Input: part model. Units: mm. Frame: model coordinates. A direction names the side the tool comes from. Coordinates: 2 decimals unless noted, no trailing zeros. Loops run counter-clockwise (first coordinate to the right, second up) from the corner with the lowest first, then second, coordinate; pieces in that order, holes last. Notation, with made-up numbers: (86.25, 21) - (93.25, 21) arc R16 cw to (93.25, 34) - close; hole circle Ø8 at (-35.75, -8.75). An arc over 180 degrees is marked (long way). Use a Markdown table: item, result. Add a question column.
1. Access query for faces 4 (the face through (35.5, -12.7, -14.9)), 5 (the face through (-38.487, 5.15, 5.616)), 6 (the face through (-7.555, -0.992, -38.486)). Directions: +Z, -Z, +X, -X, +Y, -Y. A direction counts if a zero-diameter tool reaches every point of the face in a straight line with its end or side. Return the directions, or none.
2. Draft query along Z for faces 1 (the face through (35.5, 12.7, -14.9)), 2 (the face through (11.44, -0.18, 36.34)), 3 (the face through (11.92, 0.18, 37.84)). Return one class per face: released by +Z, released by -Z, zero draft, split by the parting line, or undercut.
3. Contact query for flat-ended pins moving along their axis: P1, Ø6, axis at y = 1.5, z = -30.5, coming from the -X side; P2, Ø4, axis at x = -21, z = -28.5, coming from the +Y side; P3, Ø12, axis at x = -12, y = 9, coming from the -Z side; P4, Ø3, axis at x = -7, y = 9, coming from the +Z side. Output: stop coordinate, or through.
4. Section query B-B on z = 0. Return the cut outline in (x, y).
5. Ray query, L1, parallel to Y at x = -39, z = 0; L2, parallel to Z at x = -2.5, y = -8.75; L3, parallel to X at y = -3.75, z = 18. Return the intervals inside material, ascending. Write a range as [from, to].
6. Section query D-D on x = 14. Return the cut outline in (y, z), then the cut area to 3 significant figures.
7. Section query A-A on x = 0. Return the cut outline in (y, z).
8. Section query C-C on y = 0. Return the cut outline in (x, z), then the cut area to 3 significant figures.
```python
from build123d import *

# Parameters (mm, degrees)
SKETCH1_R           = 39.6748
SKETCH1_R_2         = 38.1
BOSS_EXTRUDE1_DEPTH = 12.7
SKETCH2_R           = 7.62
CUT_EXTRUDE1_DEPTH  = 58.527988928
SKETCH3_R           = 7.62
CUT_EXTRUDE2_DEPTH  = 58.527989088


with BuildPart() as part:
    # Sketch1 → Boss-Extrude1 (new, symmetric)
    with BuildSketch(Plane(origin=(0, 0, 0), x_dir=(1, 0, 0), z_dir=(0, 1, 0))):
        with Locations(Location((0, 0, 0), (0, 0, 270))):
            Circle(SKETCH1_R)
        with Locations(Location((0, 0, 0), (0, 0, 270))):
            Circle(SKETCH1_R_2, mode=Mode.SUBTRACT)
    extrude(amount=BOSS_EXTRUDE1_DEPTH, both=True)

    # Sketch2 → Cut-Extrude1 (cut, through all)
    with BuildSketch(Plane.XY):
        with Locations(Location((0, 0, 0), (0, 0, 90))):
            Circle(SKETCH2_R)
    extrude(amount=-CUT_EXTRUDE1_DEPTH, mode=Mode.SUBTRACT)

    # Sketch3 → Cut-Extrude2 (cut, through all)
    with BuildSketch(Plane(origin=(0, 0, 0), x_dir=(0, 0, -1), z_dir=(1, 0, 0))):
        Circle(SKETCH3_R)
    extrude(amount=-CUT_EXTRUDE2_DEPTH, mode=Mode.SUBTRACT)


solid = part.part
```
Resolved:
| question | item | result |
|---|---|---|
| 1 | face 4 | +Z, -Z, +X, -X, -Y |
| 1 | face 5 | -X |
| 1 | face 6 | -Z |
| 2 | face 1 | zero draft |
| 2 | face 2 | undercut |
| 2 | face 3 | split by the parting line |
| 3 | P1 | x = -28.6 |
| 3 | P2 | through |
| 3 | P3 | z = -39.22 |
| 3 | P4 | z = 39.29 |
| 4 | outline | (-39.67, -12.7) - (-38.1, -12.7) - (-38.1, -7.62) - (-39.67, -7.62) - close; (-39.67, 7.62) - (-38.1, 7.62) - (-38.1, 12.7) - (-39.67, 12.7) - close; (38.1, -12.7) - (39.67, -12.7) - (39.67, 12.7) - (38.1, 12.7) - close |
| 5 | L1 | [-12.7, -7.62], [7.62, 12.7] |
| 5 | L2 | [-39.6, -38.02], [38.02, 39.6] |
| 5 | L3 | [-35.36, -33.58], [33.58, 35.36] |
| 6 | outline | (-12.7, -37.12) - (12.7, -37.12) - (12.7, -35.43) - (-12.7, -35.43) - close; (-12.7, 35.43) - (12.7, 35.43) - (12.7, 37.12) - (-12.7, 37.12) - close |
| 6 | area | 85.8 mm² |
| 7 | outline | (-12.7, -39.67) - (-7.62, -39.67) - (-7.62, -38.1) - (-12.7, -38.1) - close; (-12.7, 38.1) - (12.7, 38.1) - (12.7, 39.67) - (-12.7, 39.67) - close; (7.62, -39.67) - (12.7, -39.67) - (12.7, -38.1) - (7.62, -38.1) - close |
| 8 | outline | (-38.94, -7.62) arc R39.67 ccw to (-7.62, -38.94) - (-7.62, -37.33) arc R38.1 cw to (-37.33, -7.62) - close; (-38.94, 7.62) - (-37.33, 7.62) arc R38.1 cw (long way) to (7.62, -37.33) - (7.62, -38.94) arc R39.67 ccw (long way) to start |
| 8 | area | 336 mm² |
